Could you check a few things on this model? Use its own coordinates, in mm. Face numbers are marked on the shaded views. Round coordinates to 2 decimals unless told otherwise and drop trailing zeros. Loops run counter-clockwise (first coordinate to the right, second up) from the corner with the lowest first, then second, coordinate; pieces in that order, holes last. Notation, with made-up numbers: (55, -2) -> (100, -2) arc R7 cw to (100, 10) -> close; hole circle Ø3 at (49, -7). An arc over 180 degrees is marked (long way). Write each question's results on one line, items separated by ' | '. Start each with the question number.
1) Imagine slicing it at C-C, the plane z = -10.5. List the corners of the cut face in (x, y) for me.
2) Imagine slicing it at A-A, the plane x = 0. List the corners of the cut face in (y, z) for me (3 decimals), plus the area to 3 significant figures.
3) For P1, Ø10, axis at x = -11, z = -2.5, coming from the -Y side; P2, Ø12, axis at y = 15, z = -6.5, coming from the -X side; P3, Ø1.5, axis at y = -8, z = -12.5, coming from the -X side, each with a flat end and sliding along its axis, tell me the tip position at first contact or that it passes through.
4) We'd pull the mould along Y, two halves only. Please class the marked faces 1 and 2: pulls with the +Y half, pulls with the -Y half, needs draft (parallel to the pull), parting line crosses it, or undercut.
5) If I drill on probe 1 along Y at (x, z) = (0, 1.1) (3 decimals); probe 2 along Y at (x, z) = (0, -9.75); probe 3 along Z at (x, y) = (-7, -12), over which ranges is the centre line in solid material (lowest first)?
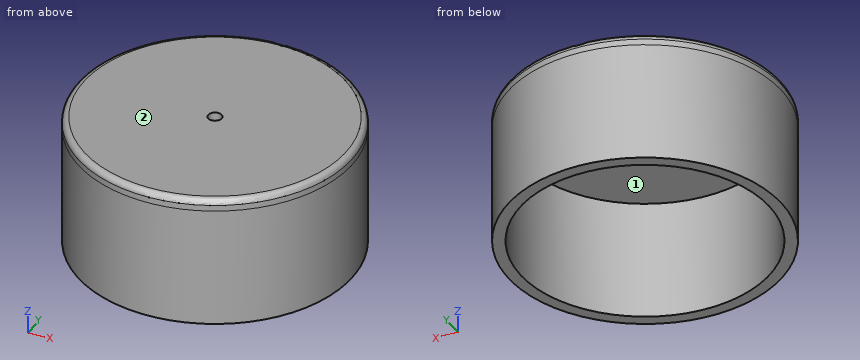
from build123d import *

# Parameters (mm, degrees)
SKETCH1_R           = 22.75
BOSS_EXTRUDE1_DEPTH = 2
BOSS_EXTRUDE2_START = 20
SKETCH2_R           = 22.75
SKETCH2_R_2         = 20.75
BOSS_EXTRUDE2_DEPTH = 20
FILLET1_R           = 1
SKETCH3_R           = 1.125
CUT_EXTRUDE1_DEPTH  = 20


with BuildPart() as part:
    # Sketch1 → Boss-Extrude1 (new body)
    with BuildSketch(Plane.XY):
        Circle(SKETCH1_R)
    extrude(amount=BOSS_EXTRUDE1_DEPTH)

    # Sketch2 → Boss-Extrude2 (add)
    with BuildSketch(Plane(origin=(0, 0, 0), x_dir=(-1, 0, 0), z_dir=(0, 0, -1)).offset(BOSS_EXTRUDE2_START)):
        Circle(SKETCH2_R)
        Circle(SKETCH2_R_2, mode=Mode.SUBTRACT)
    extrude(amount=-BOSS_EXTRUDE2_DEPTH)

    # Fillet1
    fillet1_edges = [part.edges().sort_by_distance(p)[0] for p in [
        (-22.75, 0, 2),
    ]]
    fillet(fillet1_edges, radius=FILLET1_R)

    # Sketch3 → Cut-Extrude1 (cut)
    with BuildSketch(Plane.XY.offset(2)):
        Circle(SKETCH3_R)
    extrude(amount=-CUT_EXTRUDE1_DEPTH, mode=Mode.SUBTRACT)


solid = part.part
Checked values:
1) outline: circle Ø45.5 at (0, 0); hole circle Ø41.5 at (0, 0)
2) outline: (-22.75, -20) -> (-20.75, -20) -> (-20.75, 0) -> (-1.125, 0) -> (-1.125, 2) -> (-21.75, 2) arc R1 ccw to (-22.75, 1) -> close; (1.125, 0) -> (20.75, 0) -> (20.75, -20) -> (22.75, -20) -> (22.75, 1) arc R1 ccw to (21.75, 2) -> (1.125, 2) -> close | area: 166 mm^2
3) P1: y = -21.94 | P2: x = -20.89 | P3: x = -21.56
4) face 1: undercut | face 2: needs draft
5) probe 1: -22.745 to -1.125, 1.125 to 22.745 | probe 2: -22.75 to -20.75, 20.75 to 22.75 | probe 3: 0 to 2
